Build history of the part. All positions in model axes, mm. Face numbers are marked on the shaded views. A direction names the side the tool comes from. Round coordinates to 2 decimals unless told otherwise and drop trailing zeros. Loops run counter-clockwise (first coordinate to the right, second up) from the corner with the lowest first, then second, coordinate; pieces in that order, holes last. Notation, with made-up numbers: (76, -29) - (92, -29) arc R25 cw to (92, -13) - close; hole circle Ø5 at (4.25, 45.5). An arc over 180 degrees is marked (long way). Use one line per item in the form item = value. Start each with the question number.
Q1. Drill centre lines: line 1 (Z direction, x = -6.75, y = 0); line 2 (Y direction, x = -4.75, z = -2.25); line 3 (Z direction, x = 8, y = 9). Where is each one in solid material? Low to high.
Q2. Pin check, flat tips, straight feed: pin 1 (2 mm diameter, centred on y = -4, z = -1.5, fed in from -X); pin 2 (1.5 mm diameter, centred on x = -0.5, z = 0, fed in from -Y); pin 3 (1.2 mm diameter, centred on x = -3, z = -1.5, fed in from -Y). Stop position of each tip, or through.
Q3. Saw through at D-D (z = 7). Give the cut face in (x, y).
Q4. Saw through at A-A (z = -1.25). Give the cut face in (x, y).
Q5. Saw through at B-B (y = 0). Give the cut face in (x, z).
Q6. Saw through at C-C (x = 0). Give the cut face in (y, z).
Q7. 3-axis set-ups, long thin cutter, end or side, ignore diameter. For the marked faces 1, 2, 3, 4 and 5: which of +Z, -Z, +X, -X, +Y, -Y reach the whole face in a straight line?
```python
from build123d import *

# Parameters (mm, degrees)
F0_R     = 10
F1_DEPTH = 15
F2_R     = 12.5
F3_DEPTH = 2
F4_W     = 2.5
F4_H     = 5
F4_W_2   = 5
F4_H_2   = 2.5
F5_DEPTH = 5
F6_W     = 5
F6_H     = 3
F7_DEPTH = 2
F8_R     = 1
F9_DEPTH = 3


with BuildPart() as f1:
    # F0 (on Top) → F1 (new body)
    with BuildSketch(Plane.XY):
        Circle(F0_R)
    extrude(amount=F1_DEPTH)

    # F2 (on face) → F3 (join)
    with BuildSketch(Plane.XY.offset(15)):
        Circle(F2_R)
    extrude(amount=F3_DEPTH)

    # F4 (on face) → F5 (join)
    with BuildSketch(Plane(origin=(0, 0, 0), x_dir=(1, 0, 0), z_dir=(0, 0, -1))):
        with Locations((-3.75, 0)):
            Rectangle(F4_W, F4_H)
        with Locations((0, 3.75)):
            Rectangle(F4_W_2, F4_H_2)
        Rectangle(F4_W_2, F4_H)
        with Locations((3.75, 0)):
            Rectangle(F4_W, F4_H)
        with Locations((0, -3.75)):
            Rectangle(F4_W_2, F4_H_2)
    extrude(amount=F5_DEPTH)

    # F6 (on face) → F7 (join)
    with BuildSketch(Plane.XZ.offset(5)):
        with Locations((0, -3.5)):
            Rectangle(F6_W, F6_H)
    extrude(amount=F7_DEPTH)

    # F8 (on face) → F9 (cut)
    with BuildSketch(Plane.XY.offset(17)):
        with Locations((-10.9821680997, -1.5129518582)):
            Circle(F8_R)
    extrude(amount=-F9_DEPTH, mode=Mode.SUBTRACT)


solid = f1.part
```
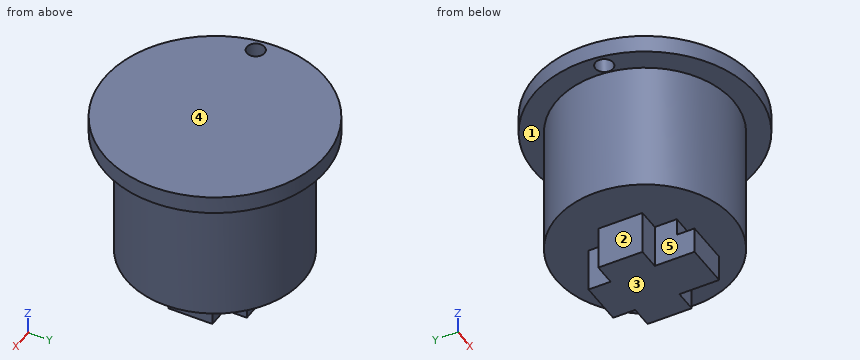
Report:
q1.line_1 = 0 to 17
q1.line_2 = -2.5 to 2.5
q1.line_3 = 15 to 17
q2.pin_1 = -2.5
q2.pin_2 = -10
q2.pin_3 = -5
q3.outline = circle Ø20 at (0, 0)
q4.outline = (-5, -2.5) - (-2.5, -2.5) - (-2.5, -5) - (2.5, -5) - (2.5, -2.5) - (5, -2.5) - (5, 2.5) - (2.5, 2.5) - (2.5, 5) - (-2.5, 5) - (-2.5, 2.5) - (-5, 2.5) - close
q5.outline = (-12.5, 15) - (-10, 15) - (-10, 0) - (-5, 0) - (-5, -5) - (5, -5) - (5, 0) - (10, 0) - (10, 15) - (12.5, 15) - (12.5, 17) - (-12.5, 17) - close
q6.outline = (-12.5, 15) - (-10, 15) - (-10, 0) - (-5, 0) - (-5, -2) - (-7, -2) - (-7, -5) - (5, -5) - (5, 0) - (10, 0) - (10, 15) - (12.5, 15) - (12.5, 17) - (-12.5, 17) - close
q7.face_1 = -Z
q7.face_2 = -Z, -X, +Y, -Y
q7.face_3 = -Z, +X, -X, +Y, -Y
q7.face_4 = +Z, +X, -X, +Y, -Y
q7.face_5 = -Z, -X, -Y
